```python
from build123d import *

# Parameters (mm, degrees)
BOSS_EXTRUDE1_DEPTH        = 41
F_10_32_TAPPED_HOLE1_D     = 4.0386
F_10_32_TAPPED_HOLE1_DEPTH = 8
F_10_32_TAPPED_HOLE1_TIP   = 1.213317848
F_10_32_TAPPED_HOLE2_D     = 4.0386
F_10_32_TAPPED_HOLE2_DEPTH = 8
F_10_32_TAPPED_HOLE2_TIP   = 1.213317848
CHAMFER1_SIZE              = 0.5


with BuildPart() as part:
    # Sketch1 → Boss-Extrude1 (new body)
    with BuildSketch(Plane(origin=(0, 0, 0), x_dir=(1, 0, 0), z_dir=(0, 1, 0))):
        Polygon((0, -5.499261314), (4.7625, -2.749630657), (4.7625, 2.749630657), (0, 5.499261314), (-4.7625, 2.749630657), (-4.7625, -2.749630657), align=None)
    extrude(amount=BOSS_EXTRUDE1_DEPTH)

    # #10-32 Tapped Hole1
    with Locations(Plane(origin=(0, 41, 0), x_dir=(1, 0, 0), z_dir=(0, 1, 0))):
        with Locations((0, 0)):
            Hole(F_10_32_TAPPED_HOLE1_D / 2, depth=F_10_32_TAPPED_HOLE1_DEPTH)
            with Locations((0, 0, -(F_10_32_TAPPED_HOLE1_DEPTH + F_10_32_TAPPED_HOLE1_TIP / 2))):  # 118° drill point
                Cone(0, F_10_32_TAPPED_HOLE1_D / 2, F_10_32_TAPPED_HOLE1_TIP, mode=Mode.SUBTRACT)

    # #10-32 Tapped Hole2
    with Locations(Plane(origin=(0, 0, 0), x_dir=(-1, 0, 0), z_dir=(0, -1, 0))):
        with Locations((0, 0)):
            Hole(F_10_32_TAPPED_HOLE2_D / 2, depth=F_10_32_TAPPED_HOLE2_DEPTH)
            with Locations((0, 0, -(F_10_32_TAPPED_HOLE2_DEPTH + F_10_32_TAPPED_HOLE2_TIP / 2))):  # 118° drill point
                Cone(0, F_10_32_TAPPED_HOLE2_D / 2, F_10_32_TAPPED_HOLE2_TIP, mode=Mode.SUBTRACT)

    # Chamfer1
    chamfer1_edges = [part.edges().sort_by_distance(p)[0] for p in [
        (2.0193, 41, 0),
        (-2.0193, 0, 0),
    ]]
    chamfer(chamfer1_edges, length=CHAMFER1_SIZE)


solid = part.part
```
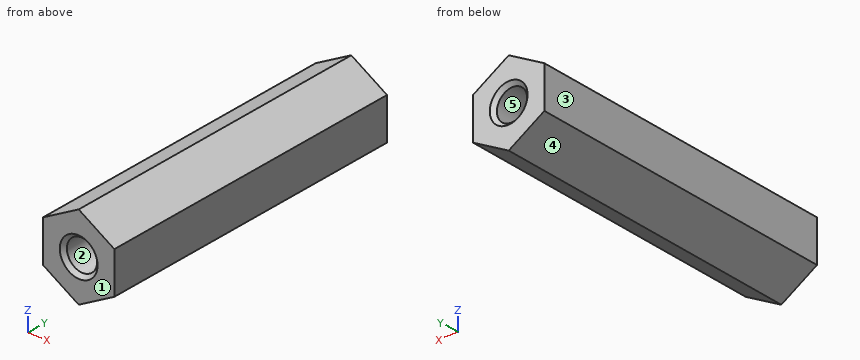
Geometry: final body of the model. Coordinates: model frame, mm. Face numbers are marked on the shaded views. A direction names the side the tool comes from. Round coordinates to 2 decimals unless told otherwise and drop trailing zeros. Order: outer loops, then holes, each group sorted by start corner. A loop starts at its lowest first (then second) coordinate and runs counter-clockwise, first axis right, second up. Notation, with made-up numbers: (64, 81.5) -> (102, 81.5) arc R9 ccw to (102, 92.5) -> close; hole circle Ø3 at (71.5, 23.5). An arc over 180 degrees is marked (long way). Use one line per item in the form item = value.
(1) Section B-B on y = 23. Return loops of the section in (x, z), and give its area (3 significant figures).
Results list:
outline = (-4.76, -2.75) -> (0, -5.5) -> (4.76, -2.75) -> (4.76, 2.75) -> (0, 5.5) -> (-4.76, 2.75) -> close
area = 78.6 mm^2
(2) Section C-C on z = 4.5. Return loops of the section in (x, y), and give its area (3 significant figures).
Results list:
outline = (-1.73, 0) -> (1.73, 0) -> (1.73, 41) -> (-1.73, 41) -> close
area = 142 mm^2
(3) Section A-A on y = 38.5. Return loops of the section in (x, z).
Results list:
outline = (-4.76, -2.75) -> (0, -5.5) -> (4.76, -2.75) -> (4.76, 2.75) -> (0, 5.5) -> (-4.76, 2.75) -> close; hole circle Ø4.04 at (0, 0)
(4) Draft query along X for the marked faces 1, 2 and 3. Return one class per face: pulls with the +X half, pulls with the -X half, needs draft (parallel to the pull), parting line crosses it, or undercut.
Results list:
face_1 = needs draft
face_2 = undercut
face_3 = pulls with the -X half
(5) First-contact query: pin 1 Ø1.5 at (y, z) = (28, 4.5) entering from -X; pin 2 Ø4.5 at (x, z) = (0, 0) entering from +Y; pin 3 Ø4.5 at (x, z) = (0, 0) entering from -Y. Flat tips, straight axial feed; report the tip coordinate or a pass-through.
Results list:
pin_1 = -3.03
pin_2 = 40.73
pin_3 = 0.27
(6) Access query for the marked faces 4 and 5. Directions: +Z, -Z, +X, -X, +Y, -Y. A direction counts if a zero-diameter tool reaches every point of the face in a straight line with its end or side. Return the directions, or none.
Results list:
face_4 = -Z, -X, +Y, -Y
face_5 = +Y
(7) Ray query, probe 1 along X at (y, z) = (37.75, 0); probe 2 along Z at (x, y) = (0, 5.25); probe 3 along Z at (x, y) = (1.5, 39). Return the intervals inside material, ascending. Write a range as [from, to].
Results list:
probe_1 = [-4.76, -2.02], [2.02, 4.76]
probe_2 = [-5.5, -2.02], [2.02, 5.5]
probe_3 = [-4.63, -1.35], [1.35, 4.63]
